Here's how the part is built. I have some questions about the finished solid (model axes, mm). Coordinates: 2 decimals unless noted, no trailing zeros. Write each loop counter-clockwise with the first axis right and the second up, starting at its lowest first coordinate (ties: lowest second). Pieces come first, ordered by that corner, then holes.
Item 1: If I drill on line 1 (Z direction, x = 10.5, y = 0); line 2 (Y direction, x = 16.75, z = 46.5); line 3 (Y direction, x = 1.75, z = -51.5), over which ranges is the centre line in solid material (lowest first)?
Item 2: If we section it at C-C (y = -51): Please give me the cut outline in (x, z), then the cut area to 3 significant figures.
Item 3: I'm going to push flat-ended pins straight in: pin 1 Ø1.5 at (x, y) = (3.5, 4) entering from +Z; pin 2 Ø8 at (x, y) = (8.5, -45.5) entering from +Z. Where does each tip first touch, or does it pass through?
Item 4: We'd pull the mould along Z, two halves only. Please class faces 1 (the face through (18, -1, -36)), 2 (the face through (8.87, 29.14, -9.18)), 3 (the face through (8.87, -17.88, 80.54)): +Z half, -Z half, draft (parallel to the pull), parting line (faces both ways), or undercut.
Item 5: If we section it at A-A (z = 0): Please give me the cut outline in (x, y), then the cut area to 3 significant figures.
Item 6: If we section it at D-D (x = 3.5): Please give me the cut outline in (y, z).
Autodesk Inventor part; units mm, degrees
ref_plane "YZ Plane" through (0, 0, 0) normal (1, 0, 0) x (0, 1, 0)
ref_plane "XZ Plane" through (0, 0, 0) normal (0, 1, 0) x (-1, 0, 0)
ref_plane "XY Plane" through (0, 0, 0) normal (0, 0, 1) x (1, 0, 0)
sketch "Sketch1" plane through (0, 0, 0) normal (0, 0, 1) x (1, 0, 0)
  line L0 (18, 82.5) -> (0, 82.5)
  line L1 (0, 82.5) -> (0, 30.55)
  line L2 (0, 30.55) -> (0, 0) construction
  line L3 (0, 0) -> (18, 0) construction
  line L4 (18, 82.5) -> (18, 30.55)
  line L5 (18, 30.55) -> (0, 30.55)
  line L6 (18, 30.55) -> (18, 0) construction
  dimension "d0" = 165
  dimension "d1" = 18
  dimension "d5" = 61.1
revolve "Revolution1" add sketch "Sketch1" angle 360 about axis through (0, 0, 0) along (1, 0, 0)
sketch "Sketch2" plane through (0, 0, 0) normal (-1, 0, 0) x (0, 0, 1)
  circle A0 centre (0, 0) radius 30.55
  line L0 (0, 62.5) -> (0, 0) construction
  circle A1 centre (0, 0) radius 82.5
  circle A2 centre (0, 0) radius 62.5 construction
  line L1 (0, 0) -> (44.1942, 44.1942) construction
  circle A3 centre (44.1942, 44.1942) radius 9
  dimension "d6" = 18
  dimension "d7" = 62.5
  dimension "d8" = 45
extrude "Extrusion1" cut sketch "Sketch2" against normal through all contours A3
pattern_circular "Circular Pattern1" count 4 over 360 about axis through (9, 0, 0) along (1, 0, 0) of "Extrusion1"
equation "\"d6\" = dd2"
equation "\"d7\" = 0.5 * k"
equation "\"d0\" = D"
equation "\"d1\" = b"
equation "\"d5\" = dd5"
equation "\"b\" = 18"
equation "\"D\" = 165"
equation "\"k\" = 125"
equation "\"dd2\" = 18"
equation "\"dd5\" = 61.1"
equation "\"Size_Designation\" = 1.2345"
properties part number "DIN 2576 Slip-On Flange for Welding Series 1 (ISO) - PN 10 50 x 60.3" material "Steel"
Answer list:
1. line 1: z = -82.5 to -30.55, 30.55 to 82.5
1. line 2: y = -68.15 to -52.89, -35.49 to 35.49, 52.89 to 68.15
1. line 3: y = -64.45 to -49.45, -38.94 to 38.94, 49.45 to 64.45
2. outline: (0, -64.85) - (18, -64.85) - (18, -50.08) - (0, -50.08) - close; (0, -38.31) - (18, -38.31) - (18, 38.31) - (0, 38.31) - close; (0, 50.08) - (18, 50.08) - (18, 64.85) - (0, 64.85) - close
2. area: 1,910 mm2
3. pin 1: stops at z = 82.44
3. pin 2: stops at z = 71.3
4. face 1: draft
4. face 2: undercut
4. face 3: parting line
5. outline: (0, -82.5) - (18, -82.5) - (18, -30.55) - (0, -30.55) - close; (0, 30.55) - (18, 30.55) - (18, 82.5) - (0, 82.5) - close
5. area: 1,870 mm2
6. outline: circle Ø165 at (0, 0); hole circle Ø18 at (-44.19, -44.19); hole circle Ø18 at (-44.19, 44.19); hole circle Ø61.1 at (0, 0); hole circle Ø18 at (44.19, -44.19); hole circle Ø18 at (44.19, 44.19)
